Design review of the part built by this model. Coordinates are the model's own, in mm. Face numbers are marked on the shaded views. Round coordinates to 2 decimals unless told otherwise and drop trailing zeros. Loops run counter-clockwise (first coordinate to the right, second up) from the corner with the lowest first, then second, coordinate; pieces in that order, holes last. Notation, with made-up numbers: (23.5, 43) - (39.5, 43) arc R19 cw to (39.5, 63) - close; hole circle Ø4 at (-38, 30.25). An arc over 180 degrees is marked (long way). Use one line per item in the form item = value. Start each with the question number.
(1) For pin 1 (10 mm diameter, centred on x = -33, z = -84.5, fed in from +Y), flat-tipped, find the tip position at first contact; note if it passes through.
(2) We need section B-B, the plane x = -96. Write out the cut boundary in (y, z), then the cut area to 3 significant figures.
(3) We need section C-C, the plane z = -20. Write out the cut boundary in (x, y), then the cut area to 3 significant figures.
(4) Wall thickness on probe 1 along Z at (x, y) = (-32, 42.05); probe 2 along Z at (x, y) = (-81, 42.5); probe 3 along X at (y, z) = (42.6, -55): over which ranges is each line inside the solid? List them lowest first. Write a range as [from, to].
(5) We need section A-A, the plane y = 42.5. Write out the cut boundary in (x, z) (3 decimals).
(6) The part is to be moulded in two halves that separate along Z. For the marked faces 1 and 2, say which applies: released by +Z, released by -Z, zero draft, split by the parting line, or undercut.
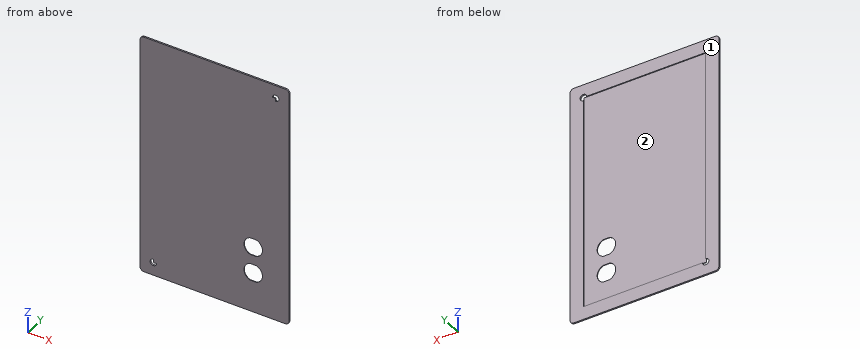
Autodesk Inventor part; units mm, degrees
ref_plane "YZ Plane" through (0, 0, 0) normal (1, 0, 0) x (0, 1, 0)
ref_plane "XZ Plane" through (0, 0, 0) normal (0, 1, 0) x (-1, 0, 0)
ref_plane "XY Plane" through (0, 0, 0) normal (0, 0, 1) x (1, 0, 0)
ref_plane "Work Plane1" through (0, 41.656, 0) normal (0, 1, 0) x (1, 0, 0)
sketch "Sketch2" plane through (0, 41.656, 0) normal (0, 1, 0) x (1, 0, 0)
  line L0 (-118.364, 207.264) -> (-10.414, 207.264)
  arc A0 (-4.064, 200.914) -> (-10.414, 207.264) centre (-10.414, 200.914) ccw
  line L1 (-4.064, 200.914) -> (-4.064, 10.414)
  arc A1 (-10.414, 4.064) -> (-4.064, 10.414) centre (-10.414, 10.414) ccw
  line L2 (-10.414, 4.064) -> (-118.364, 4.064)
  arc A2 (-124.714, 10.414) -> (-118.364, 4.064) centre (-118.364, 10.414) ccw
  line L3 (-124.714, 10.414) -> (-124.714, 200.914)
  arc A3 (-118.364, 207.264) -> (-124.714, 200.914) centre (-118.364, 200.914) ccw
  line L4 (-128.778, 208.153) -> (-128.778, 3.175)
  arc A4 (-128.778, 3.175) -> (-125.603, 0) centre (-125.603, 3.175) ccw
  line L5 (-125.603, 0) -> (-3.175, 0)
  arc A5 (-3.175, 0) -> (0, 3.175) centre (-3.175, 3.175) ccw
  line L6 (0, 3.175) -> (0, 208.153)
  arc A6 (0, 208.153) -> (-3.175, 211.328) centre (-3.175, 208.153) ccw
  line L7 (-3.175, 211.328) -> (-125.603, 211.328)
  arc A7 (-125.603, 211.328) -> (-128.778, 208.153) centre (-125.603, 208.153) ccw
  circle A8 centre (-117.348, 199.898) radius 2.794
  circle A9 centre (-11.43, 11.43) radius 2.794
  line L8 (-117.348, 199.898) -> (-11.43, 199.898)
  line L9 (-11.43, 199.898) -> (-11.43, 11.43)
  line L10 (-11.43, 11.43) -> (-117.348, 11.43)
  line L11 (-117.348, 11.43) -> (-117.348, 199.898)
  point P0 (0, 0)
extrude "Extrusion5" add sketch "Sketch2" along normal blind 1.27 contours L0 A0 L1 A1 L2 A2 L3 A3 | A7 L7 A6 L6 A5 L5 A4 L4
extrude "Extrusion6" add sketch "Sketch2" along normal blind 0.508 contours L8 L9 A9 L10 L11 A8 | A8 L11 L8 | L9 L10 A9 picked at (-115.5087, 199.6908) picked at (-13.2693, 11.6372)
sketch "Sketch3" plane through (0, 42.164, 0) normal (0, 1, 0) x (1, 0, 0)
  line L0 (-14.224, 11.43) -> (-117.348, 11.43)
  line L1 (-114.554, 199.898) -> (-11.43, 199.898)
  line L2 (-117.348, 11.43) -> (-62.992, 11.43)
  line L3 (-62.992, 11.43) -> (-62.992, 199.898)
  line L4 (-62.992, 199.898) -> (-117.348, 199.898)
  line L5 (-117.348, 199.898) -> (-117.348, 11.43)
  line L6 (-11.43, 199.898) -> (-62.992, 199.898)
  line L7 (-62.992, 199.898) -> (-62.992, 105.664)
  line L8 (-62.992, 105.664) -> (-11.43, 105.664)
  line L9 (-11.43, 105.664) -> (-11.43, 199.898)
  line L10 (-37.211, 105.664) -> (-62.992, 105.664)
  line L11 (-62.992, 105.664) -> (-62.992, 199.898)
  line L12 (-62.992, 199.898) -> (-37.211, 199.898)
  line L13 (-37.211, 199.898) -> (-37.211, 105.664)
  line L14 (-11.43, 199.898) -> (-11.43, 14.224)
  line L15 (-11.43, 199.898) -> (-37.211, 199.898)
  line L16 (-37.211, 199.898) -> (-37.211, 152.781)
  line L17 (-37.211, 152.781) -> (-11.43, 152.781)
  line L18 (-11.43, 152.781) -> (-11.43, 199.898)
  line L19 (-11.43, 105.664) -> (-24.3205, 105.664)
  line L20 (-24.3205, 105.664) -> (-24.3205, 199.898)
  line L21 (-24.3205, 199.898) -> (-11.43, 199.898)
  line L22 (-11.43, 199.898) -> (-11.43, 105.664)
  line L23 (-37.211, 176.3395) -> (-24.3205, 176.3395)
  line L24 (-24.3205, 176.3395) -> (-24.3205, 152.781)
  line L25 (-24.3205, 152.781) -> (-37.211, 152.781)
  line L26 (-37.211, 152.781) -> (-37.211, 176.3395)
  line L27 (-37.211, 105.664) -> (-24.3205, 105.664)
  line L28 (-24.3205, 105.664) -> (-24.3205, 152.781)
  line L29 (-24.3205, 152.781) -> (-37.211, 152.781)
  line L30 (-37.211, 152.781) -> (-37.211, 105.664)
  line L31 (-37.211, 129.2225) -> (-24.3205, 129.2225)
  line L32 (-24.3205, 129.2225) -> (-24.3205, 152.781)
  line L33 (-24.3205, 152.781) -> (-37.211, 152.781)
  line L34 (-37.211, 152.781) -> (-37.211, 129.2225)
  line L35 (-24.3205, 105.664) -> (-30.7657, 105.664)
  line L36 (-30.7657, 105.664) -> (-30.7657, 129.2225)
  line L37 (-30.7657, 129.2225) -> (-24.3205, 129.2225)
  line L38 (-24.3205, 129.2225) -> (-24.3205, 105.664)
  line L39 (-30.7657, 129.2225) -> (-24.3205, 129.2225)
  line L40 (-24.3205, 129.2225) -> (-24.3205, 199.898)
  line L41 (-24.3205, 199.898) -> (-30.7657, 199.898)
  line L42 (-30.7657, 199.898) -> (-30.7657, 129.2225)
  point P0 (0, 0)
sketch "Sketch4" plane through (0, 42.164, 0) normal (0, 1, 0) x (1, 0, 0)
  point P0 (0, 0)
  point P1 (-30.9206, 152.9754)
  point P2 (-30.9206, 176.1357)
hole "Hole1" at (-30.9206, 42.164, -152.9754) at (-30.9206, 42.164, -176.1357) direction (0, -1, 0) diameter 16.002 depth 8.001 tip angle 118
sketch "Sketch5" plane through (0, 42.164, 0) normal (0, 1, 0) x (1, 0, 0)
  circle A0 centre (-30.9206, 152.9754) radius 8.001
  circle A1 centre (-30.9206, 176.1357) radius 8.001
  line L0 (-30.9206, 152.9754) -> (-38.9216, 152.9754)
  line L1 (-30.9206, 152.9754) -> (-22.9196, 152.9754)
  circle A2 centre (-30.9206, 176.1357) radius 8.001
  line L2 (-38.9216, 176.1357) -> (-30.9206, 176.1357)
  line L3 (-30.9206, 176.1357) -> (-22.9196, 176.1357)
  circle A3 centre (-30.9206, 152.9754) radius 7.5057
  circle A4 centre (-30.9206, 176.1357) radius 7.5057
  line L4 (-30.9206, 152.9754) -> (-38.9216, 152.9754)
  line L5 (-38.9216, 152.9754) -> (-38.9216, 160.4811)
  line L6 (-38.9216, 160.4811) -> (-30.9206, 160.4811)
  line L7 (-30.9206, 160.4811) -> (-30.9206, 152.9754)
  line L8 (-30.9206, 152.9754) -> (-22.9196, 152.9754)
  line L9 (-22.9196, 152.9754) -> (-22.9196, 145.4697)
  line L10 (-22.9196, 145.4697) -> (-30.9206, 145.4697)
  line L11 (-30.9206, 145.4697) -> (-30.9206, 152.9754)
  line L12 (-22.9196, 145.4697) -> (-38.9216, 145.4697)
  line L13 (-38.9216, 145.4697) -> (-38.9216, 160.4811)
  line L14 (-38.9216, 160.4811) -> (-22.9196, 160.4811)
  line L15 (-22.9196, 160.4811) -> (-22.9196, 145.4697)
  line L16 (-30.9206, 176.1357) -> (-22.9196, 176.1357)
  line L17 (-22.9196, 176.1357) -> (-22.9196, 168.63)
  line L18 (-22.9196, 168.63) -> (-30.9206, 168.63)
  line L19 (-30.9206, 168.63) -> (-30.9206, 176.1357)
  line L20 (-30.9206, 176.1357) -> (-38.9216, 176.1357)
  line L21 (-38.9216, 176.1357) -> (-38.9216, 183.6414)
  line L22 (-38.9216, 183.6414) -> (-30.9206, 183.6414)
  line L23 (-30.9206, 183.6414) -> (-30.9206, 176.1357)
  line L24 (-38.9216, 183.6414) -> (-22.9196, 183.6414)
  line L25 (-22.9196, 183.6414) -> (-22.9196, 168.63)
  line L26 (-22.9196, 168.63) -> (-38.9216, 168.63)
  line L27 (-38.9216, 168.63) -> (-38.9216, 183.6414)
  circle A5 centre (-30.9206, 152.9754) radius 8.001
  circle A6 centre (-30.9206, 176.1357) radius 8.001
  line L28 (-33.692, 183.6414) -> (-28.1492, 183.6414)
  arc A7 (-28.1492, 183.6414) -> (-33.692, 183.6414) centre (-30.9206, 176.1357) ccw
  arc A8 (-33.692, 168.63) -> (-28.1492, 168.63) centre (-30.9206, 176.1357) ccw
  line L29 (-33.692, 168.63) -> (-28.1492, 168.63)
  arc A9 (-28.1492, 160.4811) -> (-33.692, 160.4811) centre (-30.9206, 152.9754) ccw
  arc A10 (-33.692, 145.4697) -> (-28.1492, 145.4697) centre (-30.9206, 152.9754) ccw
  line L30 (-33.692, 145.4697) -> (-28.1492, 145.4697)
  line L31 (-33.692, 160.4811) -> (-28.1492, 160.4811)
  point P0 (0, 0)
  dimension "d51" = 15.0114
  dimension "d52" = 15.0114
  dimension "d53" = 15.0114
  dimension "d54" = 15.0114
  dimension "d55" = 16.002
  dimension "d56" = 8.001
  dimension "d57" = 7.5057
  dimension "d58" = 7.5057
extrude "Extrusion7" add sketch "Sketch5" against normal blind 0.508 contours L14 L6 A0 | A0 L12 L10 | L24 L22 A1 | A1 L26 L18
properties part number "Lid"
Data:
q1.pin_1 = 42.16
q2.outline = (41.66, -211.33) - (42.93, -211.33) - (42.93, -199.9) - (42.16, -199.9) - (42.16, -11.43) - (42.93, -11.43) - (42.93, 0) - (41.66, 0) - close
q2.area = 125 mm^2
q3.outline = (-128.78, 41.66) - (0, 41.66) - (0, 42.93) - (-11.43, 42.93) - (-11.43, 42.16) - (-117.35, 42.16) - (-117.35, 42.93) - (-128.78, 42.93) - close
q3.area = 82.8 mm^2
q4.probe_1 = [-211.33, -183.64], [-168.63, -160.48], [-145.47, 0]
q4.probe_2 = [-211.33, -199.9], [-11.43, 0]
q4.probe_3 = [-128.78, -117.35], [-11.43, 0]
q5.outline = (-128.778, -208.153) arc R3.175 ccw to (-125.603, -211.328) - (-3.175, -211.328) arc R3.175 ccw to (0, -208.153) - (0, -3.175) arc R3.175 ccw to (-3.175, 0) - (-125.603, 0) arc R3.175 ccw to (-128.778, -3.175) - close; hole (-117.348, -197.104) arc R2.794 ccw (long way) to (-114.554, -199.898) - (-11.43, -199.898) - (-11.43, -14.224) arc R2.794 ccw (long way) to (-14.224, -11.43) - (-117.348, -11.43) - close
q6.face_1 = zero draft
q6.face_2 = undercut
